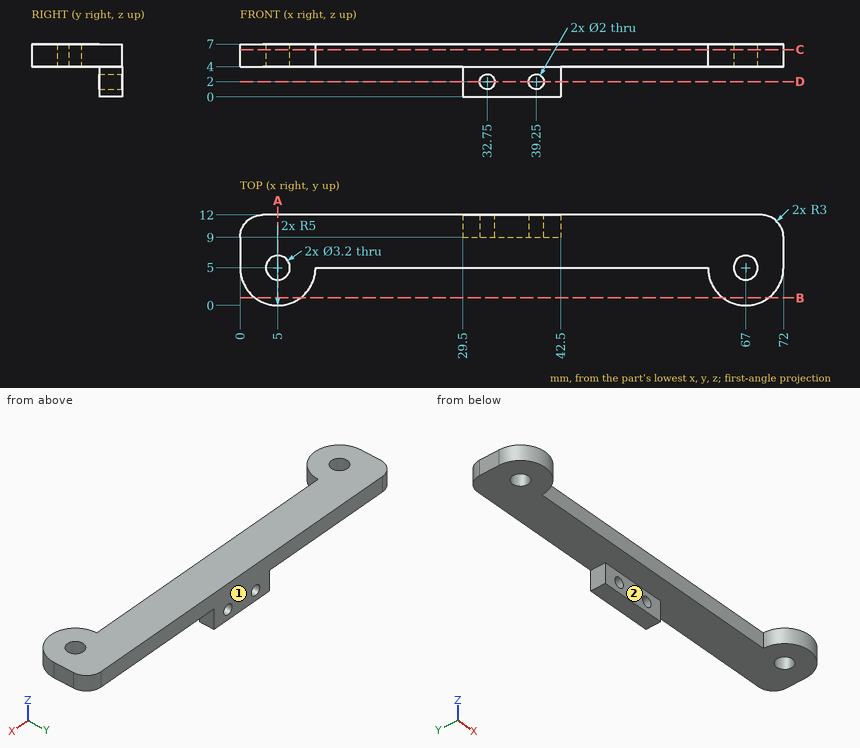
Study the drawing (mm; zero at the part's minimum x, y, z) and answer. A direction names the side the tool comes from. Give positions to 0.01 mm unless a question says otherwise; leave off trailing zeros. Write each loop counter-clockwise with the first axis right and the second up, starting at its lowest first coordinate (ties: lowest second). Pieces come first, ordered by that corner, then holes. Notation, with made-up numbers: (53.5, 81.5) - (78.5, 81.5) arc R13 cw to (78.5, 92.5) - close; hole circle Ø5 at (-8.75, 15.5). An arc over 180 degrees is marked (long way). Write item = value, one per line. Start each with the question number.
Item 1: Find section D-D (z = 2). Give the vertices of the cut face in (x, y), then the cut area to 3 significant figures.
Item 2: Find section B-B (y = 1). Give the vertices of the cut face in (x, z), then the cut area to 3 significant figures.
Item 3: Find section A-A (x = 5). Give the vertices of the cut face in (y, z), then the cut area to 3 significant figures.
Item 4: Find the intervals of material crossed by probe 1 along Y at (x, z) = (5, 6.2); probe 2 along Z at (x, y) = (39.25, 10.2); probe 3 along X at (y, z) = (5.75, 4.5), in increasing order. Write a range as [from, to].
Item 5: A tool of negligible diameter and unlimited length cuts with its end or side. For the marked faces 1 and 2, from which of +Z, -Z, +X, -X, +Y, -Y can it reach the whole face along a straight path? Write none if from no direction.
Item 6: Each of these flat-tipped pins is pushed along its axis until it touches: P1, Ø0.9, axis at y = 10, z = 2, coming from the +X side; P2, Ø3.5, axis at x = 32.5, z = 6, coming from the -Y side; P3, Ø0.9, axis at y = 11, z = 1, coming from the -X side. Where does it stop, or does it pass through?
Item 7: Find section C-C (z = 6.25). Give the vertices of the cut face in (x, y).
Response:
q1.outline = (29.5, 9) - (31.75, 9) - (31.75, 12) - (29.5, 12) - close; (33.75, 9) - (38.25, 9) - (38.25, 12) - (33.75, 12) - close; (40.25, 9) - (42.5, 9) - (42.5, 12) - (40.25, 12) - close
q1.area = 27.0 mm²
q2.outline = (2, 4) - (8, 4) - (8, 7) - (2, 7) - close; (64, 4) - (70, 4) - (70, 7) - (64, 7) - close
q2.area = 36.0 mm²
q3.outline = (0, 4) - (3.4, 4) - (3.4, 7) - (0, 7) - close; (6.6, 4) - (12, 4) - (12, 7) - (6.6, 7) - close
q3.area = 26.4 mm²
q4.probe_1 = [0, 3.4], [6.6, 12]
q4.probe_2 = [0, 1], [3, 7]
q4.probe_3 = [0, 3.59], [6.41, 65.59], [68.41, 72]
q5.face_1 = +Z, -Z, +X, -X, +Y
q5.face_2 = -Z, +X, -X, -Y
q6.P1 = 42.5
q6.P2 = 5
q6.P3 = 29.5
q7.outline = (0, 5) arc R5 ccw to (10, 5) - (62, 5) arc R5 ccw to (72, 5) - (72, 9) arc R3 ccw to (69, 12) - (3, 12) arc R3 ccw to (0, 9) - close; hole circle Ø3.2 at (5, 5); hole circle Ø3.2 at (67, 5)
